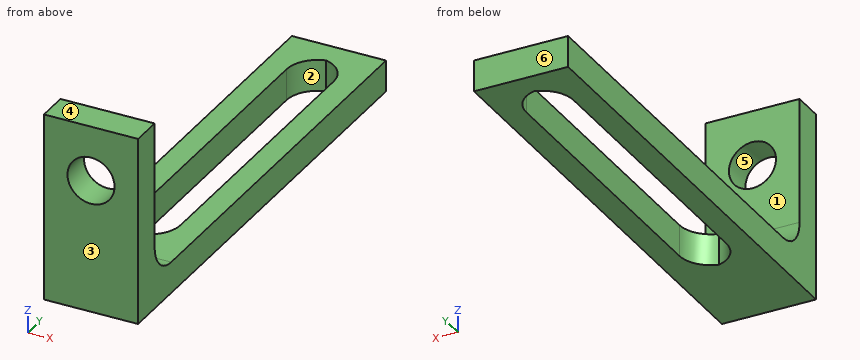
```python
from build123d import *

# Parameters (mm, degrees)
SKETCH1_W           = 6
SKETCH1_H           = 30
SKETCH1_W_2         = 3
SKETCH1_H_2         = 22.5
BOSS_EXTRUDE1_DEPTH = 2
FILLET1_R           = 2
SKETCH2_W           = 6
SKETCH2_H           = 2
BOSS_EXTRUDE2_DEPTH = 10
FILLET2_R           = 2
SKETCH3_R           = 1.5
CUT_EXTRUDE1_DEPTH  = 10


with BuildPart() as part:
    # Sketch1 → Boss-Extrude1 (new body)
    with BuildSketch(Plane.XY):
        Rectangle(SKETCH1_W, SKETCH1_H)
        with Locations((0, 2.25)):
            Rectangle(SKETCH1_W_2, SKETCH1_H_2, mode=Mode.SUBTRACT)
    extrude(amount=BOSS_EXTRUDE1_DEPTH)

    # Fillet1
    # the kernel refuses this fillet: 2 mm, written as the material it adds along each edge
    with BuildSketch(Plane(origin=(1.5, 13.5, 0), x_dir=(0, -1, 0), z_dir=(0, 0, 1)), Plane(origin=(1.5, -9, 0), x_dir=(-1, 0, 0), z_dir=(0, 0, 1)), Plane(origin=(-1.5, -9, 0), x_dir=(0, 1, 0), z_dir=(0, 0, 1))) as fillet1_piece_1:
        with BuildLine():
            CenterArc((FILLET1_R, -FILLET1_R), FILLET1_R, 90, 90)
            Line((0, -FILLET1_R), (0, 0))
            Line((0, 0), (FILLET1_R, 0))
        make_face()
    extrude(amount=2)
    with BuildSketch(Plane(origin=(-1.5, 13.5, 0), x_dir=(0, -1, 0), z_dir=(0, 0, 1))) as fillet1_piece_2:
        with BuildLine():
            CenterArc((FILLET1_R, FILLET1_R), FILLET1_R, 180, 90)
            Line((0, FILLET1_R), (0, 0))
            Line((0, 0), (FILLET1_R, 0))
        make_face()
    extrude(amount=2)

    # Sketch2 → Boss-Extrude2 (add)
    with BuildSketch(Plane.XY.offset(2)):
        with Locations((0, -14)):
            Rectangle(SKETCH2_W, SKETCH2_H)
    extrude(amount=BOSS_EXTRUDE2_DEPTH)

    # Fillet2
    fillet2_edges = [part.edges().sort_by_distance(p)[0] for p in [
        (0, -13, 2),
    ]]
    fillet(fillet2_edges, radius=FILLET2_R)

    # Sketch3 → Cut-Extrude1 (cut)
    with BuildSketch(Plane(origin=(0, -13, 0), x_dir=(1, 0, 0), z_dir=(0, 1, 0))):
        with Locations(Location((0, -8.5, 0), (0, 0, 270))):
            Circle(SKETCH3_R)
    extrude(amount=-CUT_EXTRUDE1_DEPTH, mode=Mode.SUBTRACT)


solid = part.part
```
Input: part model. Units: mm. Frame: model coordinates. Face numbers are marked on the shaded views. A direction names the side the tool comes from. Coordinates: 2 decimals unless noted, no trailing zeros. Order: outer loops, then holes, each group sorted by start corner. A loop starts at its lowest first (then second) coordinate and runs counter-clockwise, first axis right, second up. Notation, with made-up numbers: (4, 47) - (27, 47) arc R28 cw to (27, 70) - close; hole circle Ø3 at (73.25, 6). An arc over 180 degrees is marked (long way). Put each result on its own line as item: value.
1. Line query: line 1 along X through (y, z) = (-13.6, 8.5); line 2 along Y through (x, z) = (-0.3, 6.25); line 3 along Z through (x, y) = (-2.6, -4.5). Output: solid intervals per line, ascending.
Report:
line 1: x = -3 to -1.5, 1.5 to 3
line 2: y = -15 to -13
line 3: z = 0 to 2
2. Draft query along Z for the marked faces 4, 5 and 6. Return one class per face: pulls with the +Z half, pulls with the -Z half, needs draft (parallel to the pull), parting line crosses it, or undercut.
Report:
face 4: pulls with the +Z half
face 5: undercut
face 6: needs draft
3. Cut plane A-A on z = 9.5. Return the cut outline in (x, y), then the cut area to 3 significant figures.
Report:
outline: (-3, -15) - (-1.12, -15) - (-1.12, -13) - (-3, -13) - close; (1.12, -15) - (3, -15) - (3, -13) - (1.12, -13) - close
area: 7.53 mm2
4. Contact query for flat-ended pins moving along their axis: pin 1 Ø1.5 at (x, z) = (1, 8.5) entering from +Y; pin 2 Ø1.5 at (x, y) = (-2, -2) entering from +Z. Output: stop coordinate, or through.
Report:
pin 1: stops at y = -13
pin 2: stops at z = 2
5. Cut plane C-C on y = -3.5. Return the cut outline in (x, z), then the cut area to 3 significant figures.
Report:
outline: (-3, 0) - (-1.5, 0) - (-1.5, 2) - (-3, 2) - close; (1.5, 0) - (3, 0) - (3, 2) - (1.5, 2) - close
area: 6.00 mm2
6. Cut plane B-B on x = 0.9. Return the cut outline in (y, z), then the cut area to 3 significant figures.
Report:
outline: (-15, 0) - (-8.43, 0) - (-8.43, 2) - (-11, 2) arc R2 cw to (-13, 4) - (-13, 7.3) - (-15, 7.3) - close; (-15, 9.7) - (-13, 9.7) - (-13, 12) - (-15, 12) - close; (12.93, 0) - (15, 0) - (15, 2) - (12.93, 2) - close
area: 33.3 mm2
7. Cut plane D-D on x = -1.95. Return the cut outline in (y, z), then the cut area to 3 significant figures.
Report:
outline: (-15, 0) - (15, 0) - (15, 2) - (-11, 2) arc R2 cw to (-13, 4) - (-13, 12) - (-15, 12) - close
area: 80.9 mm2
8. Reachability of the marked faces 1, 2 and 3 from +Z, -Z, +X, -X, +Y, -Y: full face, straight path, thin tool, end or side. Return the list, or none.
Report:
face 1: +Z, +X, -X, +Y
face 2: +Z, -Z
face 3: +Z, -Z, +X, -X, -Y
